Part print with two shaded views. Sizes in mm from the minimum x, y, z corner. A direction names the side the tool comes from. Coordinates: 2 decimals unless noted, no trailing zeros. Loops run counter-clockwise (first coordinate to the right, second up) from the corner with the lowest first, then second, coordinate; pieces in that order, holes last.
Item 1: 3-axis set-ups, long thin cutter, end or side, ignore diameter. For the marked faces 4 and 5: which of +Z, -Z, +X, -X, +Y, -Y reach the whole face in a straight line?
Item 2: Cut at C-C (y = 40). List the corners of the cut face in (x, z), and give its area (3 significant figures).
Item 3: Cut at D-D (x = 3.5). Count the separate pieces of the cut face and the enclosed holes in it, and give its area (3 significant figures).
Item 4: Flat gauge pins, fed straight in: pin 1 (6 mm diameter, centred on y = 9.271, z = 19.05, fed in from +X); pin 2 (2.5 mm diameter, centred on x = 1.5, z = 6.5, fed in from +Y). Where does each tip first touch, or does it go through?
Item 5: Cut at A-A (y = 19.05). List the corners of the cut face in (x, z).
Item 6: Drill centre lines: line 1 along Y through (x, z) = (1.6, 29); line 2 along Z through (x, y) = (3.6, 69); line 3 along Y through (x, z) = (1.85, 19.05). Where is each one in solid material? Low to high.
Item 7: Cut at B-B (z = 19.05). List the corners of the cut face in (x, y).
Item 8: Mould opens along Y. For the marked faces 1, 2 and 3 say: released by +Y, released by -Y, zero draft, split by the parting line, or undercut.
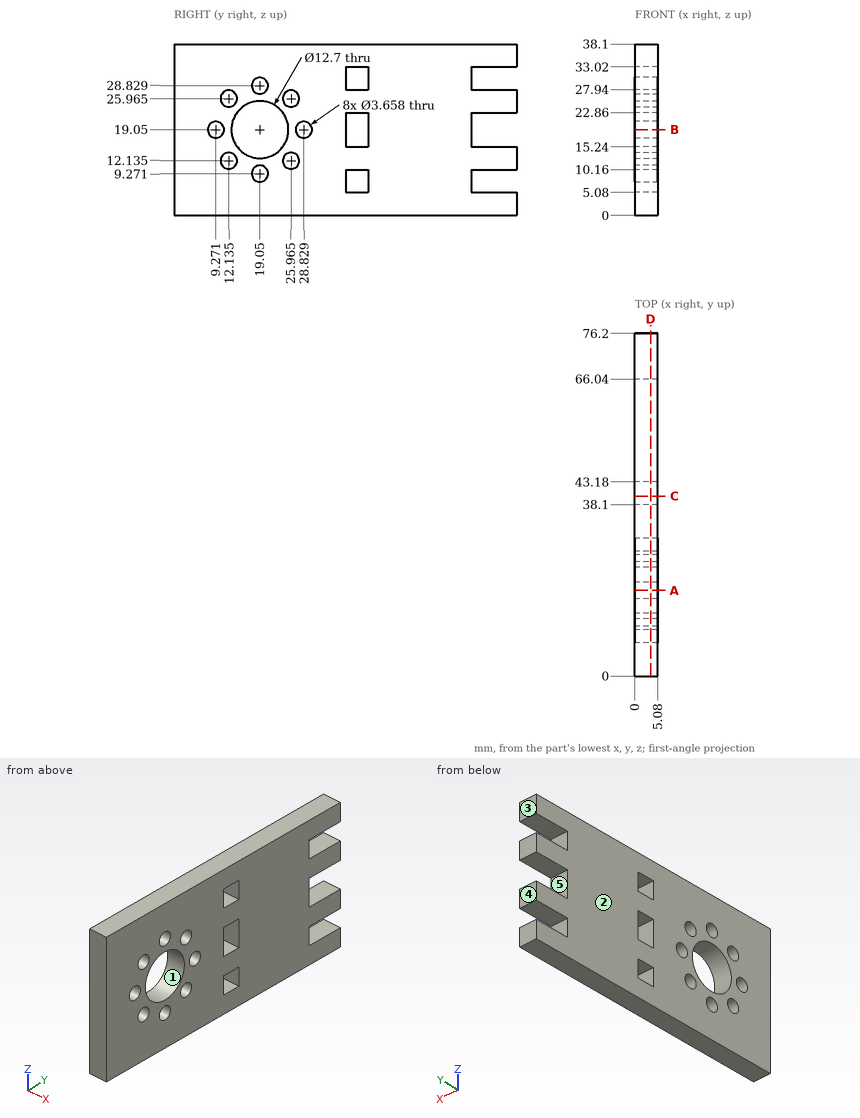
Filled sheet:
1. face 4: +Z, -Z, +X, -X, +Y
1. face 5: +X, -X, +Y
2. outline: (0, 0) - (5.08, 0) - (5.08, 5.08) - (0, 5.08) - close; (0, 10.16) - (5.08, 10.16) - (5.08, 15.24) - (0, 15.24) - close; (0, 22.86) - (5.08, 22.86) - (5.08, 27.94) - (0, 27.94) - close; (0, 33.02) - (5.08, 33.02) - (5.08, 38.1) - (0, 38.1) - close
2. area: 103 mm2
3. separate pieces: 1
3. enclosed holes: 12
3. area: 2,420 mm2
4. pin 1: stops at x = 5.08
4. pin 2: stops at y = 66.04
5. outline: (0, 0) - (5.08, 0) - (5.08, 7.44) - (0, 7.44) - close; (0, 11.1) - (5.08, 11.1) - (5.08, 12.7) - (0, 12.7) - close; (0, 25.4) - (5.08, 25.4) - (5.08, 27) - (0, 27) - close; (0, 30.66) - (5.08, 30.66) - (5.08, 38.1) - (0, 38.1) - close
6. line 1: y = 0 to 17.23, 20.87 to 38.1, 43.18 to 66.04
6. line 2: z = 0 to 5.08, 10.16 to 15.24, 22.86 to 27.94, 33.02 to 38.1
6. line 3: y = 0 to 7.44, 11.1 to 12.7, 25.4 to 27, 30.66 to 38.1, 43.18 to 66.04
7. outline: (0, 0) - (5.08, 0) - (5.08, 7.44) - (0, 7.44) - close; (0, 11.1) - (5.08, 11.1) - (5.08, 12.7) - (0, 12.7) - close; (0, 25.4) - (5.08, 25.4) - (5.08, 27) - (0, 27) - close; (0, 30.66) - (5.08, 30.66) - (5.08, 38.1) - (0, 38.1) - close; (0, 43.18) - (5.08, 43.18) - (5.08, 66.04) - (0, 66.04) - close
8. face 1: undercut
8. face 2: zero draft
8. face 3: released by +Y
